```python
from build123d import *

# Parameters (mm, degrees)
BOSS_EXTRUDE1_DEPTH = 37
SKETCH3_R           = 5
CUT_EXTRUDE1_DEPTH  = 37
SKETCH4_R           = 12
CUT_EXTRUDE2_DEPTH  = 12
SKETCH5_R           = 2
CUT_EXTRUDE3_DEPTH  = 50
SKETCH6_R           = 3
CUT_EXTRUDE4_DEPTH  = 29


with BuildPart() as part:
    # Sketch1 → Boss-Extrude1 (new body)
    with BuildSketch(Plane.XY):
        with BuildLine():
            Line((-19, 0), (-22, 0))
            Line((-22, 0), (-22, 13))
            Line((-22, 13), (-43, 13))
            Line((-43, 13), (-43, 29))
            Line((-43, 29), (-24.556058316, 29))
            ThreePointArc((-24.556058316, 29), (0, 38), (24.556058316, 29))
            Line((24.556058316, 29), (43, 29))
            Line((43, 29), (43, 13))
            Line((43, 13), (22, 13))
            Line((22, 13), (22, 0))
            Line((22, 0), (19, 0))
            ThreePointArc((19, 0), (0, 19), (-19, 0))
        make_face()
    extrude(amount=BOSS_EXTRUDE1_DEPTH)

    # Sketch3 → Cut-Extrude1 (cut)
    with BuildSketch(Plane(origin=(0, 29, 0), x_dir=(1, 0, 0), z_dir=(0, 1, 0))):
        with Locations(Location((-31, -18.5, 0), (0, 0, 270))):
            Circle(SKETCH3_R)
        with Locations(Location((31, -18.5, 0), (0, 0, 180))):
            Circle(SKETCH3_R)
    extrude(amount=-CUT_EXTRUDE1_DEPTH, mode=Mode.SUBTRACT)

    # Sketch4 → Cut-Extrude2 (cut)
    with BuildSketch(Plane(origin=(0, 29, 0), x_dir=(1, 0, 0), z_dir=(0, 1, 0))):
        with Locations((-31, -18.5)):
            Circle(SKETCH4_R)
        with Locations((31, -18.5)):
            Circle(SKETCH4_R)
    extrude(amount=CUT_EXTRUDE2_DEPTH, mode=Mode.SUBTRACT)

    # Sketch5 → Cut-Extrude3 (cut)
    with BuildSketch(Plane(origin=(0, 0, 0), x_dir=(1, 0, 0), z_dir=(0, 1, 0))):
        with Locations(Location((0, -18.5, 0), (0, 0, 90))):
            Circle(SKETCH5_R)
    extrude(amount=CUT_EXTRUDE3_DEPTH, mode=Mode.SUBTRACT)

    # Sketch6 → Cut-Extrude4 (cut)
    with BuildSketch(Plane(origin=(0, 25, 0), x_dir=(1, 0, 0), z_dir=(0, 1, 0))):
        with Locations(Location((0, -18.5, 0), (0, 0, 90))):
            Circle(SKETCH6_R)
    extrude(amount=CUT_EXTRUDE4_DEPTH, mode=Mode.SUBTRACT)


solid = part.part
```
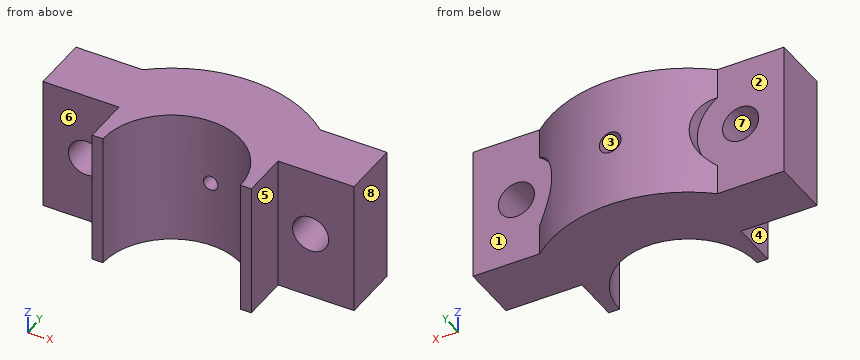
Could you check a few things on this model? Use its own coordinates, in mm. Face numbers are marked on the shaded views. A direction names the side the tool comes from. Round coordinates to 2 decimals unless told otherwise and drop trailing zeros. Write each loop counter-clockwise with the first axis right and the second up, starting at its lowest first coordinate (ties: lowest second). Pieces come first, ordered by that corner, then holes.
(1) Suppose I cut it at B-B on y = 8. Write out the boundary of the cut face in (x, z).
Findings below:
outline: (-22, 0) - (-17.23, 0) - (-17.23, 37) - (-22, 37) - close; (17.23, 0) - (22, 0) - (22, 37) - (17.23, 37) - close
(2) If I drill on probe 1 along X at (y, z) = (19, 18); probe 2 along Y at (x, z) = (-33, 28); probe 3 along Y at (x, z) = (-21.5, 17.5), over which ranges is the centre line in solid material (lowest first)?
Findings below:
probe 1: x = -43 to -35.97, -26.03 to -1.94, 1.94 to 26.03, 35.97 to 43
probe 2: y = 13 to 29
probe 3: y = 0 to 29
(3) Thinking about a two-plate mould opening in X: for the marked faces 6, 7 and 8, which applies, +X half, -X half, draft (parallel to the pull), parting line (faces both ways), or undercut?
Findings below:
face 6: draft
face 7: undercut
face 8: +X half
(4) Suppose I cut it at D-D on x = 31. Write out the boundary of the cut face in (y, z), and give its area (3 significant figures).
Findings below:
outline: (13, 0) - (29, 0) - (29, 13.5) - (13, 13.5) - close; (13, 23.5) - (29, 23.5) - (29, 37) - (13, 37) - close
area: 432 mm2
(5) Which directions (+Z, -Z, +X, -X, +Y, -Y) give clear straight access to the entire face, cutting with the end or side of a thin tool? Please do the marked faces 1, 2, 3, 4 and 5.
Findings below:
face 1: +X, +Y
face 2: -X, +Y
face 3: +Y
face 4: +Z, -Z, -X, -Y
face 5: +Z, -Z, +X, -Y
(6) For pin 1 (12 mm diameter, centred on x = -8, z = 18.5, fed in from +Y); pin 2 (2 mm diameter, centred on x = 4.5, z = 11, fed in from -Y); pin 3 (14.5 mm diameter, centred on y = 5.5, z = 11.5, fed in from -X), each with a flat end and sliding along its axis, tell me the tip position at first contact or that it passes through.
Findings below:
pin 1: stops at y = 37.93
pin 2: stops at y = 18.19
pin 3: stops at x = -22
(7) Suppose I cut it at A-A on x = 0. Write out the boundary of the cut face in (y, z).
Findings below:
outline: (19, 0) - (38, 0) - (38, 15.5) - (25, 15.5) - (25, 16.5) - (19, 16.5) - close; (19, 20.5) - (25, 20.5) - (25, 21.5) - (38, 21.5) - (38, 37) - (19, 37) - close
(8) Suppose I cut it at C-C on z = 22.5. Write out the boundary of the cut face in (x, y).
Findings below:
outline: (-43, 13) - (-34, 13) - (-34, 29) - (-43, 29) - close; (-28, 13) - (-22, 13) - (-22, 0) - (-19, 0) arc R19 cw to (19, 0) - (22, 0) - (22, 13) - (28, 13) - (28, 29) - (19.69, 29) - (19.69, 32.5) arc R38 ccw to (-19.69, 32.5) - (-19.69, 29) - (-28, 29) - close; (34, 13) - (43, 13) - (43, 29) - (34, 29) - close
